Geometry check sheet. Reference: the model listing, model coordinates, mm. Face numbers are marked on the shaded views. A direction names the side the tool comes from. Give positions to 0.01 mm unless a question says otherwise; leave off trailing zeros. Loops run counter-clockwise (first coordinate to the right, second up) from the corner with the lowest first, then second, coordinate; pieces in that order, holes last.
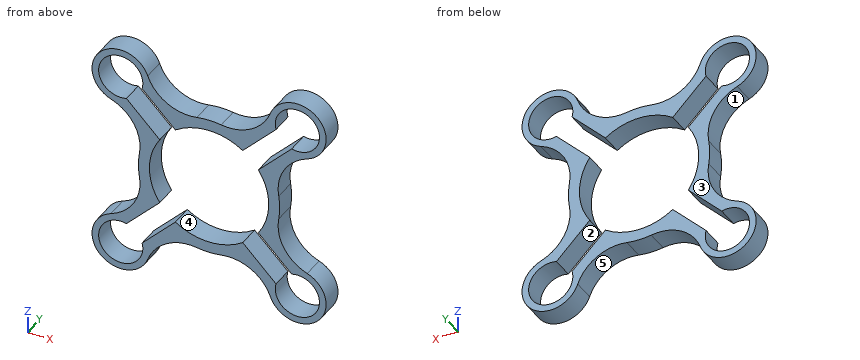
```python
from build123d import *

# Parameters (mm, degrees)
BOSS_EXTRUDE1_DEPTH = 10


with BuildPart() as part:
    # Sketch1 → Boss-Extrude1 (new body)
    with BuildSketch(Plane(origin=(0, 0, 0), x_dir=(1, 0, 0), z_dir=(0, 1, 0))):
        with BuildLine():
            ThreePointArc((-31.523820357, 5.499886369), (-32, 0), (-31.523820357, -5.499886369))
            ThreePointArc((-31.523820357, -5.499886369), (-33.916662735, -18.956279365), (-44.393071751, -27.733810979))
            ThreePointArc((-44.393071751, -27.733810979), (-49.143921292, -49.143921292), (-27.733810979, -44.393071751))
            ThreePointArc((-27.733810979, -44.393071751), (-18.956279365, -33.916662735), (-5.499886369, -31.523820357))
            ThreePointArc((-5.499886369, -31.523820357), (0, -32), (5.499886369, -31.523820357))
            ThreePointArc((5.499886369, -31.523820357), (18.956279365, -33.916662735), (27.733810979, -44.393071751))
            ThreePointArc((27.733810979, -44.393071751), (49.143921292, -49.143921292), (44.393071751, -27.733810979))
            ThreePointArc((44.393071751, -27.733810979), (33.916662735, -18.956279365), (31.523820357, -5.499886369))
            ThreePointArc((31.523820357, -5.499886369), (32, 0), (31.523820357, 5.499886369))
            ThreePointArc((31.523820357, 5.499886369), (33.916662735, 18.956279365), (44.393071751, 27.733810979))
            ThreePointArc((44.393071751, 27.733810979), (49.143921292, 49.143921292), (27.733810979, 44.393071751))
            ThreePointArc((27.733810979, 44.393071751), (18.956279365, 33.916662735), (5.499886369, 31.523820357))
            ThreePointArc((5.499886369, 31.523820357), (0, 32), (-5.499886369, 31.523820357))
            ThreePointArc((-5.499886369, 31.523820357), (-18.956279365, 33.916662735), (-27.733810979, 44.393071751))
            ThreePointArc((-27.733810979, 44.393071751), (-49.143921292, 49.143921292), (-44.393071751, 27.733810979))
            ThreePointArc((-44.393071751, 27.733810979), (-33.916662735, 18.956279365), (-31.523820357, 5.499886369))
        make_face()
        with BuildLine():
            Line((-37.363342686, 30.292274874), (-22.297196945, 15.226129133))
            ThreePointArc((-22.297196945, 15.226129133), (-27, 0), (-22.297196945, -15.226129133))
            Line((-22.297196945, -15.226129133), (-37.363342686, -30.292274874))
            ThreePointArc((-37.363342686, -30.292274874), (-47.022600949, -47.022600949), (-30.292274874, -37.363342686))
            Line((-30.292274874, -37.363342686), (-15.226129133, -22.297196945))
            ThreePointArc((-15.226129133, -22.297196945), (0, -27), (15.226129133, -22.297196945))
            Line((15.226129133, -22.297196945), (30.292274874, -37.363342686))
            ThreePointArc((30.292274874, -37.363342686), (47.022600949, -47.022600949), (37.363342686, -30.292274874))
            Line((37.363342686, -30.292274874), (22.297196945, -15.226129133))
            ThreePointArc((22.297196945, -15.226129133), (27, 0), (22.297196945, 15.226129133))
            Line((22.297196945, 15.226129133), (37.363342686, 30.292274874))
            ThreePointArc((37.363342686, 30.292274874), (47.022600949, 47.022600949), (30.292274874, 37.363342686))
            Line((30.292274874, 37.363342686), (15.226129133, 22.297196945))
            ThreePointArc((15.226129133, 22.297196945), (0, 27), (-15.226129133, 22.297196945))
            Line((-15.226129133, 22.297196945), (-30.292274874, 37.363342686))
            ThreePointArc((-30.292274874, 37.363342686), (-47.022600949, 47.022600949), (-37.363342686, 30.292274874))
        make_face(mode=Mode.SUBTRACT)
    extrude(amount=BOSS_EXTRUDE1_DEPTH)


solid = part.part
```
1) Sectioned sample at B-B on x = -25. Enter the section's corners in (y, z).
2) Sectioned sample at D-D on z = 35. Enter the section's corners in (x, y), plus the area to 3 significant figures.
3) Scan lines: line 1 along Z through (x, y) = (41, 4.25); line 2 along Z through (x, y) = (31, 0.75); line 3 along Z through (x, y) = (27.5, 3). Record each from-to range of solid material in increasing order.
4) Sectioned sample at C-C on z = -10. Enter the section's corners in (x, y), plus the area to 3 significant figures.
5) Tool access check on the marked faces 4 and 5. Record the directions out of +Z, -Z, +X, -X, +Y, -Y that give a thin tool (end or side, any length) a straight path to the whole face; none if there is none.
6) Mould release check, pull along X, two halves, no side actions. Record for the marked faces 1, 2 and 3: +X half, -X half, draft (parallel to the pull), parting line (faces both ways), or undercut.
7) Depth check by flat-ended pin: P1, Ø3, axis at x = 2.5, y = 5.5, coming from the -Z side. Enter the tip coordinate at first touch or a pass-through.
Determined:
1. outline: (0, -39.31) - (10, -39.31) - (10, -32.07) - (0, -32.07) - close; (0, -17.93) - (10, -17.93) - (10, -10.2) - (0, -10.2) - close; (0, 10.2) - (10, 10.2) - (10, 17.93) - (0, 17.93) - close; (0, 32.07) - (10, 32.07) - (10, 39.31) - (0, 39.31) - close
2. outline: (-51.97, 0) - (-48.64, 0) - (-48.64, 10) - (-51.97, 10) - close; (-27.93, 0) - (-20.63, 0) - (-20.63, 10) - (-27.93, 10) - close; (20.63, 0) - (27.93, 0) - (27.93, 10) - (20.63, 10) - close; (48.64, 0) - (51.97, 0) - (51.97, 10) - (48.64, 10) - close
2. area: 213 mm2
3. line 1: z = -52.91 to -49.9, -30.01 to -26.13, 26.13 to 30.01, 49.9 to 52.91
3. line 2: z = -49.38 to -44.41, -23.93 to 23.93, 44.41 to 49.38
3. line 3: z = -43.78 to -34.57, -20.43 to 20.43, 34.57 to 43.78
4. outline: (-31.25, 0) - (-25.08, 0) - (-25.08, 10) - (-31.25, 10) - close; (25.08, 0) - (31.25, 0) - (31.25, 10) - (25.08, 10) - close
4. area: 123 mm2
5. face 4: +Y, -Y
5. face 5: -Z, +Y, -Y
6. face 1: -X half
6. face 2: undercut
6. face 3: draft
7. P1: stops at z = -31.98
